Read the model definition and answer for the solid it produces. Units are mm, in the model's axes. A direction names the side the tool comes from. Round coordinates to 2 decimals unless told otherwise and drop trailing zeros. Order: outer loops, then holes, each group sorted by start corner. A loop starts at its lowest first (then second) coordinate and runs counter-clockwise, first axis right, second up.
from build123d import *

# Parameters (mm, degrees)
SKETCH1_W                       = 40.2
SKETCH1_H                       = 53
SKETCH1_R                       = 11.25
BOSS_EXTRUDE1_DEPTH             = 6
CBORE_FOR_M3_SBHCS1_D           = 3.4
CBORE_FOR_M3_SBHCS1_CBORE_D     = 6.7
CBORE_FOR_M3_SBHCS1_CBORE_DEPTH = 1.65
SKETCH5_W                       = 40.2
SKETCH5_H                       = 6
BOSS_EXTRUDE2_DEPTH             = 18
CUT_EXTRUDE1_REACH              = 61.473
SKETCH6_R                       = 6.45
FILLET3_R                       = 15
SKETCH8_R                       = 7.55
CUT_EXTRUDE3_DEPTH              = 3
CUT_EXTRUDE3_DIRECTION_2_REACH  = 56.194
FILLET3_OF_MIRROR1_R            = 15
FILLET4_R                       = 1
M4X0_7_TAPPED_HOLE1_D           = 3.3


with BuildPart() as part:
    # Sketch1 → Boss-Extrude1 (new body)
    with BuildSketch(Plane(origin=(0, 0, 0), x_dir=(1, 0, 0), z_dir=(0, 1, 0))):
        Rectangle(SKETCH1_W, SKETCH1_H)
        with Locations(Location((0, 0, 0), (0, 0, 270))):
            Circle(SKETCH1_R, mode=Mode.SUBTRACT)
    extrude(amount=-BOSS_EXTRUDE1_DEPTH)

    # CBORE for M3 SBHCS1 (through all)
    with Locations(Plane(origin=(0, 0, 0), x_dir=(1, 0, 0), z_dir=(0, 1, 0))):
        with Locations((-15.5, 15.5), (15.5, 15.5), (15.5, -15.5), (-15.5, -15.5)):
            CounterBoreHole(CBORE_FOR_M3_SBHCS1_D / 2, CBORE_FOR_M3_SBHCS1_CBORE_D / 2, CBORE_FOR_M3_SBHCS1_CBORE_DEPTH)

    # Sketch5 → Boss-Extrude2 (add)
    with BuildSketch(Plane(origin=(0, 0, 0), x_dir=(1, 0, 0), z_dir=(0, 1, 0))):
        with Locations((0, -23.5)):
            Rectangle(SKETCH5_W, SKETCH5_H)
    boss_extrude2 = extrude(amount=BOSS_EXTRUDE2_DEPTH)

    # Sketch6 → Cut-Extrude1 (cut, up to next)
    with BuildSketch(Plane.XY.offset(26.5), mode=Mode.PRIVATE) as cut_extrude1_sk1:
        with Locations((0, 6)):
            Circle(SKETCH6_R)
    cut_extrude1_tool1 = extrude(cut_extrude1_sk1.sketch, amount=-CUT_EXTRUDE1_REACH, mode=Mode.PRIVATE) & part.part
    cut_extrude1 = cut_extrude1_tool1.solids().sort_by_distance((0, 6, 26.5))[0]
    add(cut_extrude1, mode=Mode.SUBTRACT)

    # Fillet3
    fillet3_edges = [part.edges().sort_by_distance(p)[0] for p in [
        (20.1, 18, 23.5),
        (-20.1, 18, 23.5),
    ]]
    fillet(fillet3_edges, radius=FILLET3_R)

    # Sketch8 → Cut-Extrude3 (cut)
    with BuildSketch(Plane(origin=(0, 0, 20.5), x_dir=(-1, 0, 0), z_dir=(0, 0, -1))):
        with Locations(Location((0, 6, 0), (0, 0, 232.627116603))):
            Circle(SKETCH8_R)
    cut_extrude3 = extrude(amount=-CUT_EXTRUDE3_DEPTH, mode=Mode.SUBTRACT)

    # Sketch8 → Cut-Extrude3 direction 2 (cut, up to next)
    with BuildSketch(Plane(origin=(0, 0, 20.5), x_dir=(-1, 0, 0), z_dir=(0, 0, -1)), mode=Mode.PRIVATE) as cut_extrude3_direction_2_sk1:
        with Locations(Location((0, 6, 0), (0, 0, 232.627116603))):
            Circle(SKETCH8_R)
    cut_extrude3_direction_2_tool1 = extrude(cut_extrude3_direction_2_sk1.sketch, amount=CUT_EXTRUDE3_DIRECTION_2_REACH, mode=Mode.PRIVATE) & part.part
    cut_extrude3_direction_2 = cut_extrude3_direction_2_tool1.solids().sort_by_distance((0, 6, 20.5))[0]
    add(cut_extrude3_direction_2, mode=Mode.SUBTRACT)

    # Mirror1: Boss-Extrude2, Cut-Extrude1, Cut-Extrude3, Cut-Extrude3 direction 2 across plane
    add(boss_extrude2.mirror(Plane.XY))
    add(cut_extrude1.mirror(Plane.XY), mode=Mode.SUBTRACT)
    add(cut_extrude3.mirror(Plane.XY), mode=Mode.SUBTRACT)
    add(cut_extrude3_direction_2.mirror(Plane.XY), mode=Mode.SUBTRACT)

    # Fillet3 of Mirror1
    fillet3_of_mirror1_edges = [part.edges().sort_by_distance(p)[0] for p in [
        (20.1, 18, -23.5),
        (-20.1, 18, -23.5),
    ]]
    fillet(fillet3_of_mirror1_edges, radius=FILLET3_OF_MIRROR1_R)

    # Fillet4
    fillet4_edges = [part.edges().sort_by_distance(p)[0] for p in [
        (20.1, 1.5, 20.5),
        (15.706601718, 13.606601718, 20.5),
        (0, 18, 20.5),
        (-15.706601718, 13.606601718, 20.5),
        (20.1, 1.5, -20.5),
        (15.706601718, 13.606601718, -20.5),
        (0, 18, -20.5),
        (-15.706601718, 13.606601718, -20.5),
        (20.1, -1.5, -26.5),
        (15.706601718, 13.606601718, -26.5),
        (0, 18, -26.5),
        (-15.706601718, 13.606601718, -26.5),
        (20.1, -1.5, 26.5),
        (15.706601718, 13.606601718, 26.5),
        (0, 18, 26.5),
        (-15.706601718, 13.606601718, 26.5),
        (20.1, 0, 0),
        (-20.1, 0, 0),
        (0, -6, 26.5),
        (0, -6, -26.5),
        (-20.1, 1.5, 20.5),
        (-20.1, 1.5, -20.5),
        (-20.1, -1.5, -26.5),
        (-20.1, -1.5, 26.5),
    ]]
    fillet(fillet4_edges, radius=FILLET4_R)

    # M4x0.7 Tapped Hole1 (through all)
    with Locations(Plane(origin=(0, -6, 0), x_dir=(-1, 0, 0), z_dir=(0, -1, 0))):
        with Locations((-8, 17.5), (-8, -17.5)):
            Hole(M4X0_7_TAPPED_HOLE1_D / 2)


solid = part.part
Q1. For a pull along Z with two mould halves and no side action, classify faces 1 (the face through (-12, 0, 0)), 2 (the face through (0, 18, -23)), 3 (the face through (-7, 5, -23.5)), 4 (the face through (-5, 1, 26.5)) as released by +Z, released by -Z, zero draft, split by the parting line, or undercut.
Outcome:
face 1: undercut
face 2: zero draft
face 3: undercut
face 4: released by +Z
Q2. Flat-ended cylindrical pins translate along their axes: pin 1 (5.5 mm diameter, centred on x = 16.5, z = -17, fed in from +Y); pin 2 (4 mm diameter, centred on x = 15.5, z = -15.5, fed in from +Y). Find the tip coordinate at first contact, or state that the pin passes through.
Outcome:
pin 1: stops at y = 0
pin 2: stops at y = -1.65
Q3. Straight lines are drawn through the part: probe 1 along X at (y, z) = (-4.9, 15.5); probe 2 along Z at (x, y) = (15.5, -3.45); probe 3 along Z at (x, y) = (-13, 0.75). For each, find the intervals that lie inside material, in ascending order.
Outcome:
probe 1: x = -20.1 to -17.2, -13.8 to 13.8, 17.2 to 20.1
probe 2: z = -26.5 to -17.2, -13.8 to 13.8, 17.2 to 26.5
probe 3: z = -26.5 to -20.5, 20.5 to 26.5
Q4. For faces 5 (the face through (6.15, 7.94, -25.02)), 6 (the face through (-15.94, -0.81, 12.18)), 7 (the face through (12, 0, 0)), determine the directions among +Z, -Z, +X, -X, +Y, -Y from which every point of the face is accessible in a straight line to the end or side of a thin tool.
Outcome:
face 5: +Z, -Z
face 6: +Y
face 7: +X, -X, +Y
Q5. A cutting plane is placed at B-B, the plane y = 1. Give the number of separate pieces and of enclosed holes in the cut face, plus the area to 3 significant figures.
Outcome:
separate pieces: 4
enclosed holes: 0
area: 364 mm2
Q6. A cutting plane is placed at A-A, the plane z = 0. Give the vertices of the cut face in (x, y), plus the area to 3 significant figures.
Outcome:
outline: (-20.1, -6) - (-11.25, -6) - (-11.25, 0) - (-19.1, 0) arc R1 ccw to (-20.1, -1) - close; (11.25, -6) - (20.1, -6) - (20.1, -1) arc R1 ccw to (19.1, 0) - (11.25, 0) - close
area: 106 mm2
